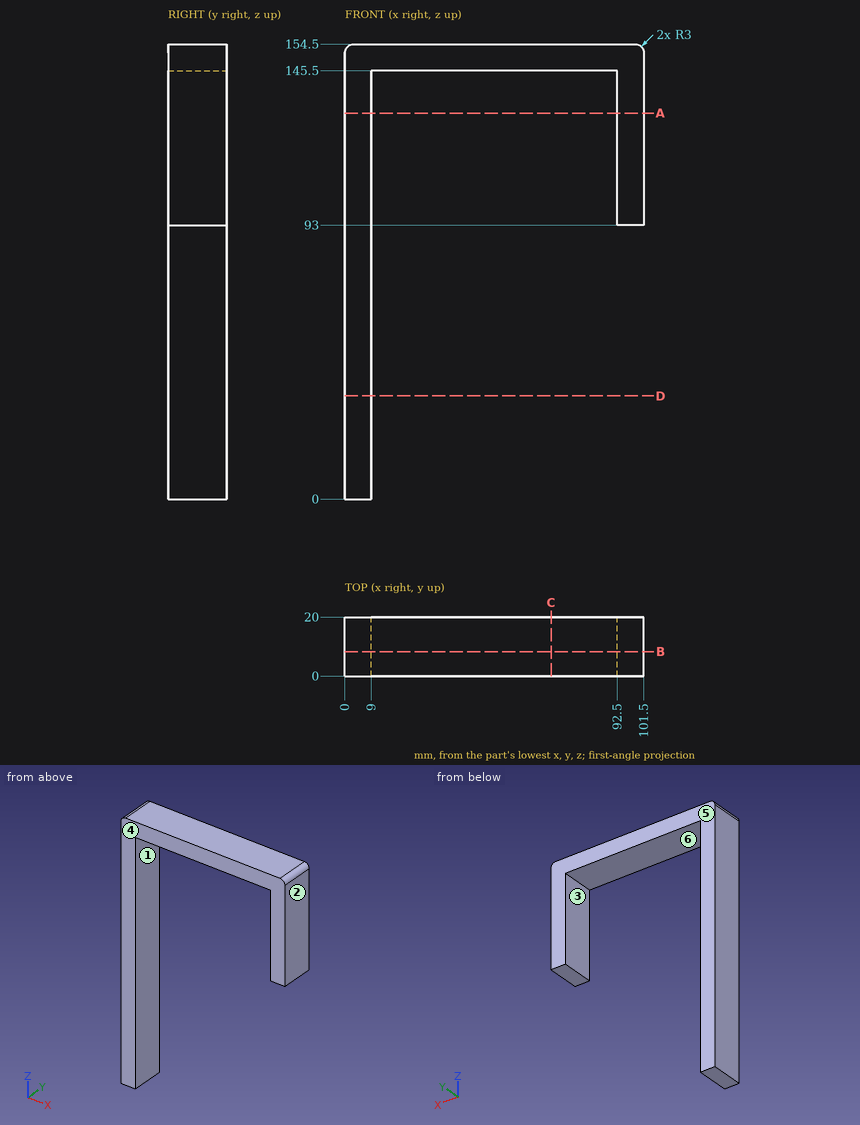
Answer from the drawing. Dimensions are ordinates in mm from the lowest x, y and z of the part. A direction names the side the tool comes from. Round coordinates to 2 decimals unless told otherwise and drop trailing zeros. Loops run counter-clockwise (first coordinate to the right, second up) from the corner with the lowest first, then second, coordinate; pieces in that order, holes last.
(1) The mould has two halves that part along X. Classify the marked faces 1, 2, 3 and 4: pulls with the +X half, pulls with the -X half, needs draft (parallel to the pull), parting line crosses it, or undercut.
Computed values:
face 1: undercut
face 2: pulls with the +X half
face 3: undercut
face 4: needs draft
(2) Find the intervals of material crossed by L1, parallel to X at y = 5.25, z = 121; L2, parallel to Z at x = 65.5, y = 14.5; L3, parallel to X at y = 3.25, z = 79.5, in increasing order.
Computed values:
L1: x = 0 to 9, 92.5 to 101.5
L2: z = 145.5 to 154.5
L3: x = 0 to 9
(3) The part is cut by section A-A, the plane z = 131. Give the vertices of the cut face in (x, y).
Computed values:
outline: (0, 0) - (9, 0) - (9, 20) - (0, 20) - close; (92.5, 0) - (101.5, 0) - (101.5, 20) - (92.5, 20) - close
(4) For the marked faces 5 and 6, determine the directions among +Z, -Z, +X, -X, +Y, -Y from which every point of the face is accessible in a straight line to the end or side of a thin tool.
Computed values:
face 5: +Z, -Z, +X, -X, +Y
face 6: -Z, +Y, -Y
(5) Each of these flat-tipped pins is pushed along its axis until it touches: P1, Ø6, axis at y = 4, z = 60, coming from the +X side; P2, Ø7, axis at x = 95, y = 11, coming from the -Z side; P3, Ø6, axis at x = 48.5, y = 6, coming from the -Z side. Where does it stop, or does it pass through?
Computed values:
P1: stops at x = 9
P2: stops at z = 93
P3: stops at z = 145.5
(6) The part is cut by section C-C, the plane x = 70. Give the vertices of the cut face in (y, z).
Computed values:
outline: (0, 145.5) - (20, 145.5) - (20, 154.5) - (0, 154.5) - close
(7) The part is cut by section D-D, the plane z = 35. Give the vertices of the cut face in (x, y), and give its area (3 significant figures).
Computed values:
outline: (0, 0) - (9, 0) - (9, 20) - (0, 20) - close
area: 180 mm2
(8) The part is cut by section B-B, the plane y = 8.25. Give the vertices of the cut face in (x, z).
Computed values:
outline: (0, 0) - (9, 0) - (9, 145.5) - (92.5, 145.5) - (92.5, 93) - (101.5, 93) - (101.5, 151.5) arc R3 ccw to (98.5, 154.5) - (3, 154.5) arc R3 ccw to (0, 151.5) - close
